Input: dimensioned drawing with shaded views. Units: mm. Origin: part minimum x, y, z. Round coordinates to 2 decimals unless told otherwise and drop trailing zeros. Order: outer loops, then holes, each group sorted by start corner. A loop starts at its lowest first (then second) coordinate and runs counter-clockwise, first axis right, second up.
Item 1: First-contact query: pin 1 (8 mm diameter, centred on y = 5, z = 12.5, fed in from -X); pin 2 (6.5 mm diameter, centred on y = 9.94, z = 27.5, fed in from +X); pin 3 (17.5 mm diameter, centred on x = 13, z = 14, fed in from +Y) (1 decimal); pin 4 (5 mm diameter, centred on x = 12, y = 8, fed in from +Z). Flat tips, straight axial feed; report the tip coordinate or a pass-through.
Item 2: Line query: L1, parallel to X at y = 2.05, z = 16.04 (1 decimal); L2, parallel to Z at x = 3.5, y = 1.2 (1 decimal); L3, parallel to X at y = 2.75, z = 28.5. Output: solid intervals per line, ascending.
Item 3: Cut plane C-C on z = 2.54. Output: boundary loops of the cut face in (x, y) (1 decimal), then the cut area to 3 significant figures.
Item 4: Cut plane A-A on z = 8. Output: boundary loops of the cut face in (x, y).
Item 5: Cut plane B-B on x = 31.5. Output: boundary loops of the cut face in (y, z) (1 decimal).
Item 6: Mould query, pull axis X, two halves, no side actions, for the marked faces 1, 2 and 3. Classes: released by +X, released by -X, zero draft, split by the parting line, or undercut.
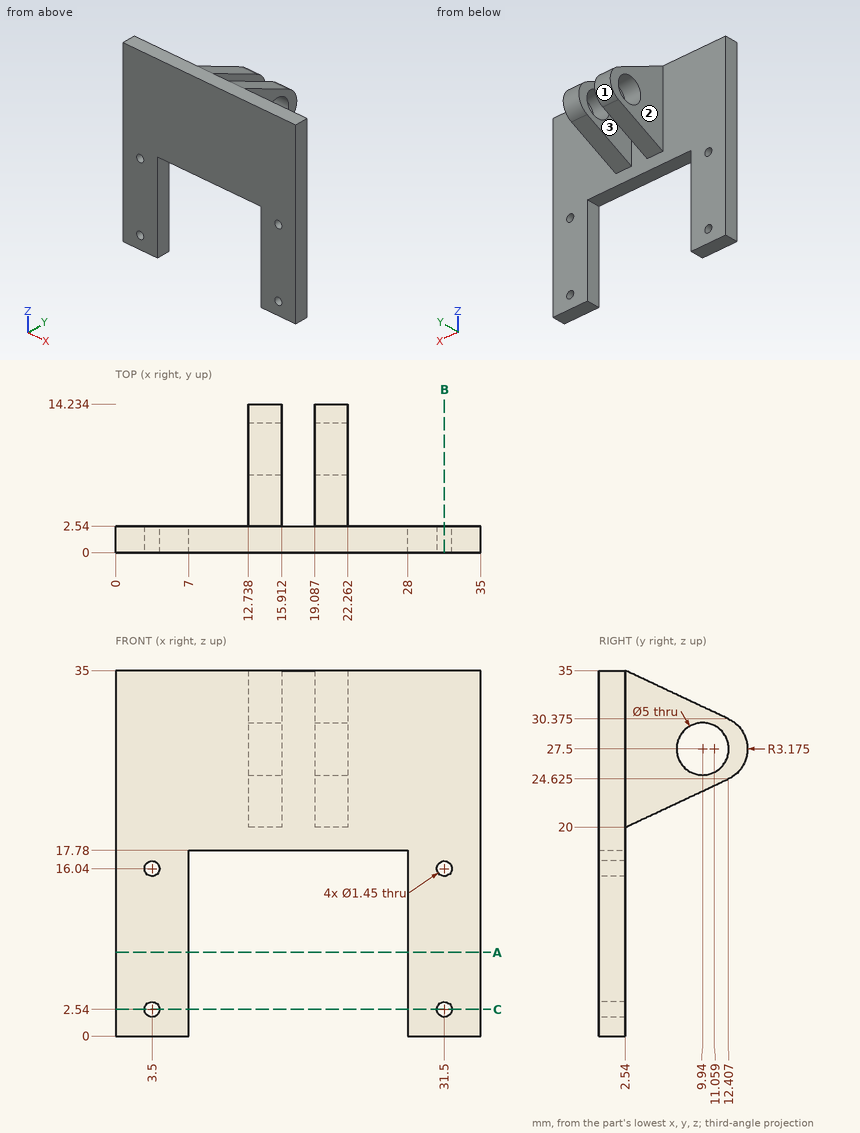
From the geometry:
1. pin 1: stops at x = 0
1. pin 2: stops at x = 22.26
1. pin 3: stops at y = 8.4
1. pin 4: stops at z = 33.56
2. L1: x = 0 to 2.8, 4.2 to 7, 28 to 30.8, 32.2 to 35
2. L2: z = 0 to 1.8, 3.3 to 15.3, 16.8 to 35
2. L3: x = 12.74 to 15.91, 19.09 to 22.26
3. outline: (0, 0) - (2.8, 0) - (2.8, 2.5) - (0, 2.5) - close; (4.2, 0) - (7, 0) - (7, 2.5) - (4.2, 2.5) - close; (28, 0) - (30.8, 0) - (30.8, 2.5) - (28, 2.5) - close; (32.2, 0) - (35, 0) - (35, 2.5) - (32.2, 2.5) - close
3. area: 28.2 mm2
4. outline: (0, 0) - (7, 0) - (7, 2.54) - (0, 2.54) - close; (28, 0) - (35, 0) - (35, 2.54) - (28, 2.54) - close
5. outline: (0, 0) - (2.5, 0) - (2.5, 1.8) - (0, 1.8) - close; (0, 3.3) - (2.5, 3.3) - (2.5, 15.3) - (0, 15.3) - close; (0, 16.8) - (2.5, 16.8) - (2.5, 35) - (0, 35) - close
6. face 1: zero draft
6. face 2: released by -X
6. face 3: undercut
